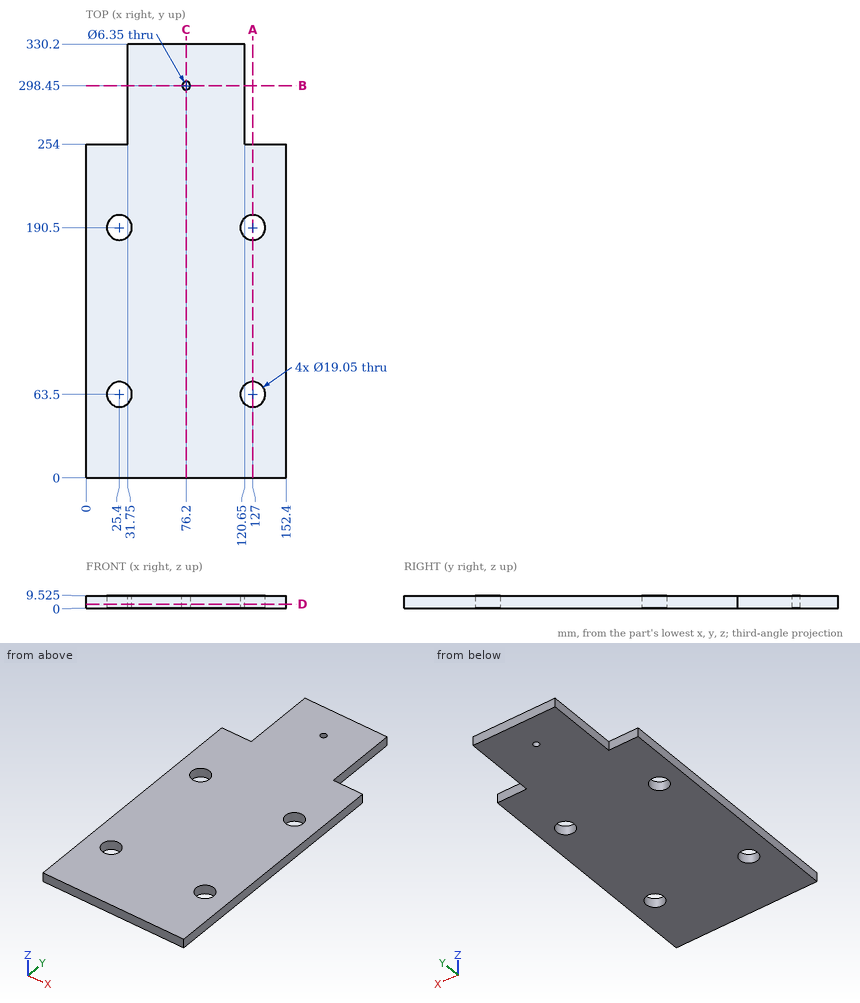
Study the drawing (mm; zero at the part's minimum x, y, z) and answer. Coordinates: 2 decimals unless noted, no trailing zeros. Order: outer loops, then holes, each group sorted by start corner. A loop starts at its lowest first (then second) coordinate and runs counter-clockwise, first axis right, second up. Notation, with made-up numbers: M 55.25,-6.75 L 92.25,-6.75 A14 cw 92.25,12.25 Z; hole C 25.25,54 d1. An arc over 180 degrees is marked long. Use CSV: the item, a comma, the result in double quotes.
Q1. Section C-C (x = 76.2) is taken. Determine the outline of the cut face in (y, z) (3 decimals), then the cut area to 3 significant figures.
Here are the results:
outline,"M 0,0 L 295.275,0 L 295.275,9.525 L 0,9.525 Z; M 301.625,0 L 330.2,0 L 330.2,9.525 L 301.625,9.525 Z"
area,"3,080 mm2"
Q2. Section D-D (z = 3.25) is taken. Determine the outline of the cut face in (x, y) (3 decimals), then the cut area to 3 significant figures.
Here are the results:
outline,"M 0,0 L 152.4,0 L 152.4,254 L 120.65,254 L 120.65,330.2 L 31.75,330.2 L 31.75,254 L 0,254 Z; hole C 25.4,63.5 d19.05; hole C 25.4,190.5 d19.05; hole C 76.2,298.45 d6.35; hole C 127,63.5 d19.05; hole C 127,190.5 d19.05"
area,"44,300 mm2"
Q3. Section B-B (y = 298.45) is taken. Determine the outline of the cut face in (x, z) (3 decimals).
Here are the results:
outline,"M 31.75,0 L 73.025,0 L 73.025,9.525 L 31.75,9.525 Z; M 79.375,0 L 120.65,0 L 120.65,9.525 L 79.375,9.525 Z"
Q4. Given pin 1 Ø3 at (y, z) = (273.5, 3.5) entering from -X; pin 2 Ø4 at (x, y) = (76.2, 298.45) entering from -Z; pin 3 Ø5 at (x, z) = (11, 6.5) entering from +Y, each flat-ended and moving along its own axis, determine where each tip first touches the part or whether it passes through.
Here are the results:
pin 1,"x = 31.75"
pin 2,"through"
pin 3,"y = 254"
Q5. Straight lines are drawn through the part: L1, parallel to Y at x = 25.4, z = 3.25 (3 decimals); L2, parallel to Y at x = 121.5, z = 6.25; L3, parallel to X at y = 193.5, z = 0.5. For each, find the intervals that lie inside material, in ascending order.
Here are the results:
L1,"0 to 53.975, 73.025 to 180.975, 200.025 to 254"
L2,"0 to 55.72, 71.28 to 182.72, 198.28 to 254"
L3,"0 to 16.36, 34.44 to 117.96, 136.04 to 152.4"
Q6. Section A-A (x = 127) is taken. Determine the outline of the cut face in (y, z) (3 decimals).
Here are the results:
outline,"M 0,0 L 53.975,0 L 53.975,9.525 L 0,9.525 Z; M 73.025,0 L 180.975,0 L 180.975,9.525 L 73.025,9.525 Z; M 200.025,0 L 254,0 L 254,9.525 L 200.025,9.525 Z"
